Geometry check sheet. Reference: the model listing, model coordinates, mm. Face numbers are marked on the shaded views. Give positions to 0.01 mm unless a question says otherwise; leave off trailing zeros. Order: outer loops, then holes, each group sorted by start corner. A loop starts at its lowest first (then second) coordinate and runs counter-clockwise, first axis right, second up. Notation, with made-up numbers: M 51.25,34 L 72.25,34 A33 cw 72.25,71 Z; hole C -13.5,-21 d7. An arc over 180 degrees is marked long. Put each result on its own line as item: value. Start each with the question number.
Q1. Section check B-B on x = 241.3. Record the cut outline in (y, z), then the cut area to 3 significant figures.
Q2. Material ranges on L1, parallel to X at y = 1.8, z = 10; L2, parallel to Z at x = 290, y = 0.8; L3, parallel to X at y = 1.65, z = 84, recorded low to high.
Q3. Go/stop test with a flat-tipped pin: pin 1 (7 mm diameter, centred on x = 133.5, z = 74, fed in from +Y). Record where the tip stops, or that it passes through.
Q4. Mould release check, pull along Z, two halves, no side actions. Record for the marked faces 1 and 2: +Z half, -Z half, draft (parallel to the pull), parting line (faces both ways), or undercut.
Q5. Section check A-A on z = 75. Record the cut outline in (x, y).
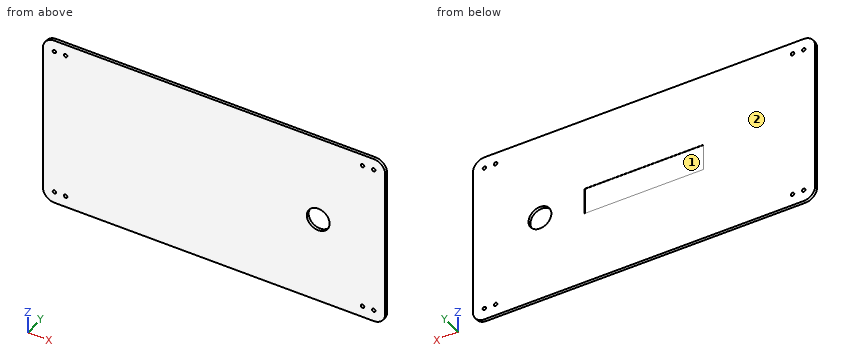
```python
from build123d import *

# Parameters (mm, degrees)
SKETCH1_W               = 300
SKETCH1_H               = 150
BOSS_EXTRUDE1_DEPTH     = 2.6
FILLET1_R               = 10
SKETCH6_R               = 1.5
CUT_EXTRUDE6_DEPTH      = 2.6
MIRROR6_COPY_1_SKETCH_R = 1.5
MIRROR6_COPY_1_DEPTH    = 2.6
SKETCH23_R              = 1.524
CUT_EXTRUDE16_DEPTH     = 2.59999988
MIRROR8_COPY_1_SKETCH_R = 1.524
MIRROR8_COPY_1_DEPTH    = 2.59999988
SKETCH15_R              = 10
CUT_EXTRUDE19_DEPTH     = 336.420273687
SKETCH25_W              = 104.14
SKETCH25_H              = 22.86
CUT_EXTRUDE20_DEPTH     = 0.254


with BuildPart() as part:
    # Sketch1 → Boss-Extrude1 (new body)
    with BuildSketch(Plane(origin=(0, 0, 0), x_dir=(1, 0, 0), z_dir=(0, 1, 0))):
        with Locations((150, -75)):
            Rectangle(SKETCH1_W, SKETCH1_H)
    extrude(amount=BOSS_EXTRUDE1_DEPTH)

    # Fillet1
    fillet1_edges = [part.edges().sort_by_distance(p)[0] for p in [
        (0, 1.3, 0),
        (300, 1.3, 0),
        (300, 1.3, 150),
        (0, 1.3, 150),
    ]]
    fillet(fillet1_edges, radius=FILLET1_R)

    # Sketch6 → Cut-Extrude6 (cut)
    with BuildSketch(Plane.XZ):
        with Locations(Location((290, 10, 0), (0, 0, 270))):
            Circle(SKETCH6_R)
    cut_extrude6 = extrude(amount=-CUT_EXTRUDE6_DEPTH, mode=Mode.SUBTRACT)

    # Mirror5: Cut-Extrude6 across plane
    add(cut_extrude6.mirror(Plane(origin=(150, 0, 0), x_dir=(0, 0, 1), z_dir=(1, 0, 0))), mode=Mode.SUBTRACT)

    # Mirror6: Cut-Extrude6 across plane
    add(cut_extrude6.mirror(Plane.XY.offset(75)), mode=Mode.SUBTRACT)

    # Mirror6 copy 1 sketch → Mirror6 copy 1 (cut)
    with BuildSketch(Plane(origin=(300, 0, 150), x_dir=(-1, 0, 0), z_dir=(0, -1, 0))):
        with Locations(Location((290, 10, 0), (0, 0, 270))):
            Circle(MIRROR6_COPY_1_SKETCH_R)
    extrude(amount=-MIRROR6_COPY_1_DEPTH, mode=Mode.SUBTRACT)

    # Sketch23 → Cut-Extrude16 (cut)
    with BuildSketch(Plane(origin=(0, 2.6, 0), x_dir=(1, 0, 0), z_dir=(0, 1, 0))):
        with Locations(Location((19.812, -9.906, 0), (0, 0, 270))):
            Circle(SKETCH23_R)
    cut_extrude16 = extrude(amount=-CUT_EXTRUDE16_DEPTH, mode=Mode.SUBTRACT)

    # Mirror7: Cut-Extrude16 across plane
    add(cut_extrude16.mirror(Plane(origin=(150, 0, 0), x_dir=(0, 0, 1), z_dir=(1, 0, 0))), mode=Mode.SUBTRACT)

    # Mirror8: Cut-Extrude16 across plane
    add(cut_extrude16.mirror(Plane.XY.offset(75)), mode=Mode.SUBTRACT)

    # Mirror8 copy 1 sketch → Mirror8 copy 1 (cut)
    with BuildSketch(Plane(origin=(300, 2.6, 150), x_dir=(-1, 0, 0), z_dir=(0, 1, 0))):
        with Locations(Location((19.812, -9.906, 0), (0, 0, 270))):
            Circle(MIRROR8_COPY_1_SKETCH_R)
    extrude(amount=-MIRROR8_COPY_1_DEPTH, mode=Mode.SUBTRACT)

    # Sketch15 → Cut-Extrude19 (cut, through all)
    with BuildSketch(Plane.XZ):
        with Locations(Location((241.3, 75, 0), (0, 0, 270))):
            Circle(SKETCH15_R)
    extrude(amount=-CUT_EXTRUDE19_DEPTH, mode=Mode.SUBTRACT)

    # Sketch25 → Cut-Extrude20 (cut)
    with BuildSketch(Plane(origin=(0, 2.6, 0), x_dir=(1, 0, 0), z_dir=(0, 1, 0))):
        with Locations((150, -75)):
            Rectangle(SKETCH25_W, SKETCH25_H)
    extrude(amount=-CUT_EXTRUDE20_DEPTH, mode=Mode.SUBTRACT)


solid = part.part
```
Results found:
1. outline: M 0,0 L 2.6,0 L 2.6,65 L 0,65 Z; M 0,85 L 2.6,85 L 2.6,150 L 0,150 Z
1. area: 338 mm^2
2. L1: x = 0 to 8.5, 11.5 to 18.29, 21.33 to 278.67, 281.71 to 288.5, 291.5 to 300
2. L2: z = 0 to 8.5, 11.5 to 138.5, 141.5 to 150
2. L3: x = 0 to 236.94, 245.66 to 300
3. pin 1: stops at y = 2.35
4. face 1: undercut
4. face 2: draft
5. outline: M 0,0 L 231.3,0 L 231.3,2.6 L 202.07,2.6 L 202.07,2.35 L 97.93,2.35 L 97.93,2.6 L 0,2.6 Z; M 251.3,0 L 300,0 L 300,2.6 L 251.3,2.6 Z
